Work out the finished part from the listing and answer in its coordinate system (mm). Coordinates: 2 decimals unless noted, no trailing zeros. Write each loop counter-clockwise with the first axis right and the second up, starting at its lowest first coordinate (ties: lowest second). Pieces come first, ordered by that corner, then holes. Notation, with made-up numbers: M 17.5,-15.75 L 24.5,-15.75 A20 cw 24.5,-1.75 Z; hole C 51.5,54 d9. An arc over 180 degrees is marked long. Answer as CSV lines item,"result". Start each with the question number.
(1) Find the intervals of material crossed by L1, parallel to Y at x = 26.5, z = 1.6; L2, parallel to X at y = -42, z = 1.2; L3, parallel to Y at x = -25.5, z = 1.55, in increasing order. Write a range as [from, to].
(2) A cutting plane is placed at A-A on x = 26.5. Give the vertices of the cut face in (y, z).
(3) A cutting plane is placed at B-B on z = 2. Count the separate pieces of the cut face and the enclosed holes in it, then the cut area to 3 significant figures.
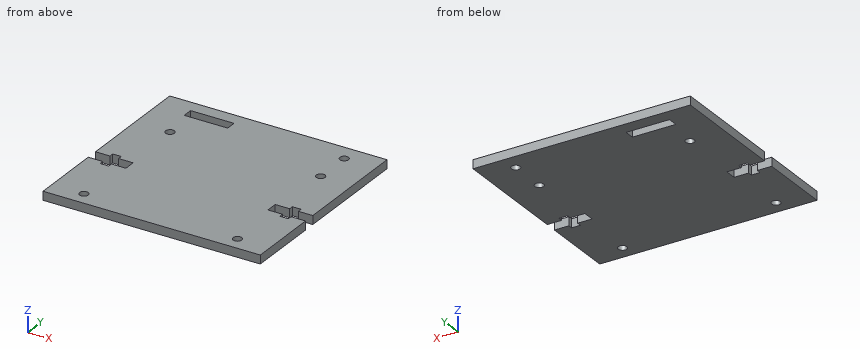
from build123d import *

# Parameters (mm, degrees)
ESQUISSE1_R        = 1.5
ESQUISSE1_W        = 15
ESQUISSE1_H        = 3.5
BOSS_EXTRU_1_DEPTH = 3


with BuildPart() as part:
    # Esquisse1 → Boss.-Extru.1 (new body)
    with BuildSketch(Plane.XY):
        Polygon((-37.5, -21.774747117), (-37.5, -46.774747117), (37.5, -46.774747117), (37.5, -21.774747117), (32.5, -21.774747117), (32.5, -23.274747117), (29.5, -23.274747117), (29.5, -21.774747117), (24.5, -21.774747117), (24.5, -17.774747117), (29.5, -17.774747117), (29.5, -16.274747117), (32.5, -16.274747117), (32.5, -17.774747117), (37.5, -17.774747117), (37.5, 23.225252883), (-37.5, 23.225252883), (-37.5, -17.774747117), (-32.5, -17.774747117), (-32.5, -16.274747117), (-29.5, -16.274747117), (-29.5, -17.774747117), (-24.5, -17.774747117), (-24.5, -21.774747117), (-29.5, -21.774747117), (-29.5, -23.274747117), (-32.5, -23.274747117), (-32.5, -21.774747117), align=None)
        with Locations((-26.5, -41.774747117)):
            Circle(ESQUISSE1_R, mode=Mode.SUBTRACT)
        with Locations((26.5, -41.774747117)):
            Circle(ESQUISSE1_R, mode=Mode.SUBTRACT)
        with Locations((-25.5, 4.225252883)):
            Circle(ESQUISSE1_R, mode=Mode.SUBTRACT)
        with Locations((-20, 16.975252883)):
            Rectangle(ESQUISSE1_W, ESQUISSE1_H, mode=Mode.SUBTRACT)
        with Locations((26.5, 4.225252883)):
            Circle(ESQUISSE1_R, mode=Mode.SUBTRACT)
        with Locations((26.5, 17.225252883)):
            Circle(ESQUISSE1_R, mode=Mode.SUBTRACT)
    extrude(amount=BOSS_EXTRU_1_DEPTH)


solid = part.part
Here are the results:
1,L1,"y = [-46.77, -43.27], [-40.27, -21.77], [-17.77, 2.73], [5.73, 15.73], [18.73, 23.23]"
1,L2,"x = [-37.5, -27.98], [-25.02, 25.02], [27.98, 37.5]"
1,L3,"y = [-46.77, -42.89], [-40.66, -21.77], [-17.77, 2.73], [5.73, 15.23], [18.73, 23.23]"
2,outline,"M -46.77,0 L -43.27,0 L -43.27,3 L -46.77,3 Z; M -40.27,0 L -21.77,0 L -21.77,3 L -40.27,3 Z; M -17.77,0 L 2.73,0 L 2.73,3 L -17.77,3 Z; M 5.73,0 L 15.73,0 L 15.73,3 L 5.73,3 Z; M 18.73,0 L 23.23,0 L 23.23,3 L 18.73,3 Z"
3,separate pieces,"1"
3,enclosed holes,"6"
3,area,"5,040 mm^2"
